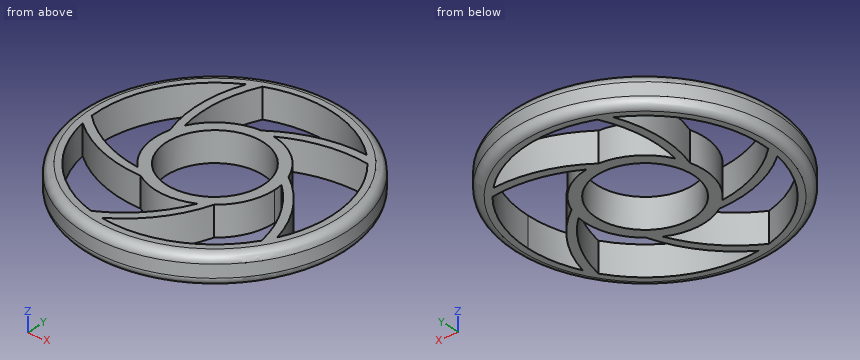
from build123d import *

# Parameters (mm, degrees)
F0_R     = 31
F0_R_2   = 11.35
F1_DEPTH = 7
F2_R     = 2


# Not quite as in the source:
# - a feature names something its author has since deleted; it is built from what else it names


with BuildPart() as f1:
    # F0 (on Top) → F1 (new body)
    with BuildSketch(Plane.XY):
        Circle(F0_R)
        with BuildLine():
            ThreePointArc((21.1666938057, 17.5562260562), (25.8682631776, 9.3318251254), (27.5, 0))
            ThreePointArc((27.5, 0), (26.7912185144, -6.2032741767), (24.7014101446, -12.0867835617))
            ThreePointArc((24.7014101446, -12.0867835617), (24.0053577694, -13.4161394731), (23.237831293, -14.7055498639))
            ThreePointArc((23.237831293, -14.7055498639), (11.5349334666, -24.9638801055), (-3.8620587477, -27.2274586076))
            ThreePointArc((-3.8620587477, -27.2274586076), (-5.3414433626, -26.9762670287), (-6.8049242418, -26.6447556953))
            ThreePointArc((-6.8049242418, -26.6447556953), (-20.1775703762, -18.6846368365), (-27.0882937172, -4.740711285))
            ThreePointArc((-27.0882937172, -4.740711285), (-27.3065513165, -3.2561104403), (-27.4435057653, -1.7618147778))
            ThreePointArc((-27.4435057653, -1.7618147778), (-24.0053577694, 13.4161394731), (-12.8794274668, 24.2975379026))
            ThreePointArc((-12.8794274668, 24.2975379026), (-11.5349334666, 24.9638801055), (-10.1560950916, 25.5558942808))
            ThreePointArc((-10.1560950916, 25.5558942808), (5.3414433626, 26.9762670287), (19.1283697872, 19.7574155518))
            ThreePointArc((19.1283697872, 19.7574155518), (20.1775703762, 18.6846368365), (21.1666938057, 17.5562260562))
        make_face(mode=Mode.SUBTRACT)
        with BuildLine():
            ThreePointArc((13.0616927236, 5.0390657066), (8.8208386376, 10.871651472), (2.2395865353, 13.8197052122))
            ThreePointArc((2.2395865353, 13.8197052122), (0.7460119592, 13.9801096618), (-0.7561512494, 13.9795649177))
            ThreePointArc((-0.7561512494, 13.9795649177), (-7.6137659317, 11.7486411273), (-12.4512503955, 6.400497136))
            ThreePointArc((-12.4512503955, 6.400497136), (-13.065344019, 5.0295910037), (-13.5290198963, 3.6007805605))
            ThreePointArc((-13.5290198963, 3.6007805605), (-13.5264047658, -3.6105919337), (-9.9348824822, -9.8639804372))
            ThreePointArc((-9.9348824822, -9.8639804372), (-8.8208386376, -10.871651472), (-7.605242881, -11.7541601453))
            ThreePointArc((-7.605242881, -11.7541601453), (-0.7460119592, -13.9801096618), (6.3111553473, -12.4967723106))
            ThreePointArc((6.3111553473, -12.4967723106), (7.6137659317, -11.7486411273), (8.8287213032, -10.8652510395))
            ThreePointArc((8.8287213032, -10.8652510395), (12.6412439705, -6.016556397), (14, 0))
            ThreePointArc((14, 0), (13.9587870879, 1.0734351561), (13.8353909951, 2.1405503996))
            ThreePointArc((13.8353909951, 2.1405503996), (13.5264047658, 3.6105919337), (13.0616927236, 5.0390657066))
        make_face()
        Circle(F0_R_2, mode=Mode.SUBTRACT)
        with BuildLine():
            ThreePointArc((2.2395865353, 13.8197052122), (11.3945871221, 17.2509213593), (21.1666938057, 17.5562260562))
            ThreePointArc((21.1666938057, 17.5562260562), (20.1775703762, 18.6846368365), (19.1283697872, 19.7574155518))
            ThreePointArc((19.1283697872, 19.7574155518), (8.6718028957, 18.6384798978), (-0.7561512494, 13.9795649177))
            ThreePointArc((-0.7561512494, 13.9795649177), (0.7460119592, 13.9801096618), (2.2395865353, 13.8197052122))
        make_face()
        with BuildLine():
            ThreePointArc((-12.4512503955, 6.400497136), (-12.8854801062, 16.1677242016), (-10.1560950916, 25.5558942808))
            ThreePointArc((-10.1560950916, 25.5558942808), (-11.5349334666, 24.9638801055), (-12.8794274668, 24.2975379026))
            ThreePointArc((-12.8794274668, 24.2975379026), (-15.046513294, 14.0069816897), (-13.5290198963, 3.6007805605))
            ThreePointArc((-13.5290198963, 3.6007805605), (-13.065344019, 5.0295910037), (-12.4512503955, 6.400497136))
        make_face()
        with BuildLine():
            ThreePointArc((-9.9348824822, -9.8639804372), (-19.3582517891, -7.258718282), (-27.4435057653, -1.7618147778))
            ThreePointArc((-27.4435057653, -1.7618147778), (-27.3065513165, -3.2561104403), (-27.0882937172, -4.740711285))
            ThreePointArc((-27.0882937172, -4.740711285), (-17.9710595236, -9.9816891338), (-7.605242881, -11.7541601453))
            ThreePointArc((-7.605242881, -11.7541601453), (-8.8208386376, -10.871651472), (-9.9348824822, -9.8639804372))
        make_face()
        with BuildLine():
            ThreePointArc((-6.8049242418, -26.6447556953), (-5.3414433626, -26.9762670287), (-3.8620587477, -27.2274586076))
            ThreePointArc((-3.8620587477, -27.2274586076), (3.9397876946, -20.1760048395), (8.8287213032, -10.8652510395))
            ThreePointArc((8.8287213032, -10.8652510395), (7.6137659317, -11.7486411273), (6.3111553473, -12.4967723106))
            ThreePointArc((6.3111553473, -12.4967723106), (0.9214225378, -20.6538588146), (-6.8049242418, -26.6447556953))
        make_face()
        with BuildLine():
            ThreePointArc((23.237831293, -14.7055498639), (24.0053577694, -13.4161394731), (24.7014101446, -12.0867835617))
            ThreePointArc((24.7014101446, -12.0867835617), (20.4059822273, -2.4877676142), (13.0616927236, 5.0390657066))
            ThreePointArc((13.0616927236, 5.0390657066), (13.5264047658, 3.6105919337), (13.8353909951, 2.1405503996))
            ThreePointArc((13.8353909951, 2.1405503996), (19.9277222355, -5.5060684643), (23.237831293, -14.7055498639))
        make_face()
    extrude(amount=F1_DEPTH)

    # F2
    f2_edges = [f1.edges().sort_by_distance(p)[0] for p in [
        (-31, 0, 7),
        (-31, 0, 0),
    ]]
    fillet(f2_edges, radius=F2_R)


solid = f1.part
The model under review builds one solid part; all positions refer to its coordinate system, in mm. Coordinates: 2 decimals unless noted, no trailing zeros. Write each loop counter-clockwise with the first axis right and the second up, starting at its lowest first coordinate (ties: lowest second). Pieces come first, ordered by that corner, then holes. Notation, with made-up numbers: (-37, -25.75) -> (7, -25.75) arc R10 cw to (7, -18.75) -> close; hole circle Ø7 at (-31, 56.5). An arc over 180 degrees is marked (long way). Answer in a Markdown table with one row per item.
1. We need section C-C, the plane y = 21. Give the number of separate pieces and of enclosed holes in the cut face, and give its area (3 significant figures).
Answers below:
| item | result |
|---|---|
| separate pieces | 3 |
| enclosed holes | 0 |
| area | 80.6 mm^2 |
2. Clearance check with flat-ended pins moving along their axes: pin 1 Ø2 at (x, z) = (-25, 4.5) entering from -Y; pin 2 Ø2 at (y, z) = (-17.5, 3) entering from -X; pin 3 Ø3 at (x, z) = (-16.5, 3.5) entering from +Y. State where each tip first meets the part, or that it passes through.
Answers below:
| item | result |
|---|---|
| pin 1 | stops at y = -19.62 |
| pin 2 | stops at x = -26.24 |
| pin 3 | stops at y = 27.13 |
3. We need section A-A, the plane z = 4.25. State the section outline as (x, y) points, and give its area (3 significant figures).
Answers below:
| item | result |
|---|---|
| outline | circle Ø62 at (0, 0); hole (-27.44, -1.76) arc R30 ccw to (-9.93, -9.86) arc R14 cw to (-13.53, 3.6) arc R30 cw to (-12.88, 24.3) arc R27.5 ccw to start; hole (-27.09, -4.74) arc R27.5 ccw to (-6.8, -26.64) arc R30 ccw to (6.31, -12.5) arc R14 cw to (-7.61, -11.75) arc R30 cw to start; hole (-12.45, 6.4) arc R14 cw to (-0.76, 13.98) arc R30 cw to (19.13, 19.76) arc R27.5 ccw to (-10.16, 25.56) arc R30 ccw to start; hole circle Ø22.7 at (0, 0); hole (-3.86, -27.23) arc R27.5 ccw to (23.24, -14.71) arc R30 ccw to (13.84, 2.14) arc R14 cw to (8.83, -10.87) arc R30 cw to start; hole (2.24, 13.82) arc R14 cw to (13.06, 5.04) arc R30 cw to (24.7, -12.09) arc R27.5 ccw to (21.17, 17.56) arc R30 ccw to start |
| area | 1,050 mm^2 |
4. We need section B-B, the plane x = 0. State the section outline as (y, z) points.
Answers below:
| item | result |
|---|---|
| outline | (-31, 2) arc R2 ccw to (-29, 0) -> (-27.5, 0) -> (-27.5, 7) -> (-29, 7) arc R2 ccw to (-31, 5) -> close; (-24.36, 0) -> (-21.6, 0) -> (-21.6, 7) -> (-24.36, 7) -> close; (-14, 0) -> (-11.35, 0) -> (-11.35, 7) -> (-14, 7) -> close; (11.35, 0) -> (14.52, 0) -> (14.52, 7) -> (11.35, 7) -> close; (27.5, 0) -> (29, 0) arc R2 ccw to (31, 2) -> (31, 5) arc R2 ccw to (29, 7) -> (27.5, 7) -> close |
5. Wall thickness on probe 1 along Y at (x, z) = (16.5, 5.75) (3 decimals); probe 2 along Y at (x, z) = (9, 6.25); probe 3 along X at (y, z) = (-24.5, 0.5): over which ranges is each line inside the solid? List them lowest first. Write a range as [from, to].
Answers below:
| item | result |
|---|---|
| probe 1 | y = [-26.071, -22], [-0.592, 2.165], [17.811, 19.825], [22, 26.071] |
| probe 2 | y = [-29.21, -25.99], [-10.72, -6.92], [6.92, 10.72], [16.68, 18.73], [25.99, 29.21] |
| probe 3 | x = [-17.87, -12.49], [-3.41, -0.16], [12.49, 17.87] |
